Here's how the part is built. I have some questions about the finished solid (model axes, mm). Face numbers are marked on the shaded views. Round coordinates to 2 decimals unless told otherwise and drop trailing zeros. Order: outer loops, then holes, each group sorted by start corner. A loop starts at its lowest first (then second) coordinate and runs counter-clockwise, first axis right, second up.
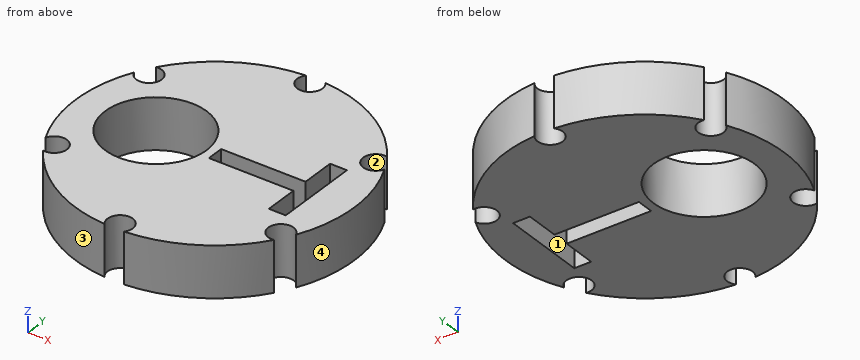
```python
from build123d import *

# Parameters (mm, degrees)
SKETCH1_R           = 16.5
BOSS_EXTRUDE1_DEPTH = 6
SKETCH2_R           = 1.5
CUT_EXTRUDE1_DEPTH  = 25.093567606
SKETCH3_R           = 6
CUT_EXTRUDE2_DEPTH  = 25.065971427
CUT_EXTRUDE3_DEPTH  = 25.065971427


with BuildPart() as part:
    # Sketch1 → Boss-Extrude1 (new body)
    with BuildSketch(Plane.XY):
        Circle(SKETCH1_R)
    extrude(amount=BOSS_EXTRUDE1_DEPTH)

    # Sketch2 → Cut-Extrude1 (cut, through all)
    with BuildSketch(Plane.XY.offset(6)):
        with Locations((0, 15.5)):
            Circle(SKETCH2_R)
        with Locations((13.423393759, 7.75)):
            Circle(SKETCH2_R)
        with Locations((13.423393759, -7.75)):
            Circle(SKETCH2_R)
        with Locations((0, -15.5)):
            Circle(SKETCH2_R)
        with Locations((-13.423393759, -7.75)):
            Circle(SKETCH2_R)
        with Locations((-13.423393759, 7.75)):
            Circle(SKETCH2_R)
    extrude(amount=-CUT_EXTRUDE1_DEPTH, mode=Mode.SUBTRACT)

    # Sketch3 → Cut-Extrude2 (cut, through all)
    with BuildSketch(Plane.XY.offset(6)):
        with Locations((-7, 0)):
            Circle(SKETCH3_R)
    extrude(amount=-CUT_EXTRUDE2_DEPTH, mode=Mode.SUBTRACT)

    # Sketch5 → Cut-Extrude3 (cut, through all)
    with BuildSketch(Plane.XY.offset(6)):
        Polygon((12, 5), (10, 5), (10, 1), (0, 1), (0, -1), (10, -1), (10, -5), (12, -5), align=None)
    extrude(amount=-CUT_EXTRUDE3_DEPTH, mode=Mode.SUBTRACT)


solid = part.part
```
1. I need wall thicknesses on probe 1 along X at (y, z) = (3, 3.9); probe 2 along Y at (x, z) = (12.5, 0.45); probe 3 along X at (y, z) = (7.75, 1.95). Which ranges of each line are inside material? Lowest first, please.
Evaluation:
probe 1: x = -16.22 to -12.2, -1.8 to 10, 12 to 16.22
probe 2: y = -10.77 to -8.93, -6.57 to 6.57, 8.93 to 10.77
probe 3: x = -11.92 to 11.92
2. I'm going to push flat-ended pins straight in: P1, Ø0.6, axis at x = 11, z = 2, coming from the +Y side; P2, Ø3, axis at x = 11.5, z = 5, coming from the +Y side. Where does each tip first touch, or does it pass through?
Evaluation:
P1: stops at y = 12.56
P2: stops at y = 13.12
3. If we section it at A-A, the plane y = 0: Write out the boundary of the cut face in (x, z), and give its area (3 significant figures).
Evaluation:
outline: (-16.5, 0) - (-13, 0) - (-13, 6) - (-16.5, 6) - close; (-1, 0) - (0, 0) - (0, 6) - (-1, 6) - close; (12, 0) - (16.5, 0) - (16.5, 6) - (12, 6) - close
area: 54.0 mm2
4. If we section it at D-D, the plane y = 15.5: Write out the boundary of the cut face in (x, z).
Evaluation:
outline: (-5.66, 0) - (-1.5, 0) - (-1.5, 6) - (-5.66, 6) - close; (1.5, 0) - (5.66, 0) - (5.66, 6) - (1.5, 6) - close
5. If we mould it in two halves opening along X, with no side actions, what happens to the marked faces 1, 2, 3 and 4? For each: released by +X, released by -X, zero draft, split by the parting line, or undercut.
Evaluation:
face 1: undercut
face 2: undercut
face 3: released by -X
face 4: released by +X
6. If we section it at C-C, the plane z = 4.05: Write out the boundary of the cut face in (x, y).
Evaluation:
outline: (-14.83, -7.23) arc R1.5 cw (long way) to (-13.68, -9.23) arc R16.5 ccw to (-1.15, -16.46) arc R1.5 cw (long way) to (1.15, -16.46) arc R16.5 ccw to (13.68, -9.23) arc R1.5 cw (long way) to (14.83, -7.23) arc R16.5 ccw to (14.83, 7.23) arc R1.5 cw (long way) to (13.68, 9.23) arc R16.5 ccw to (1.15, 16.46) arc R1.5 cw (long way) to (-1.15, 16.46) arc R16.5 ccw to (-13.68, 9.23) arc R1.5 cw (long way) to (-14.83, 7.23) arc R16.5 ccw to start; hole circle Ø12 at (-7, 0); hole (0, -1) - (10, -1) - (10, -5) - (12, -5) - (12, 5) - (10, 5) - (10, 1) - (0, 1) - close
7. If we section it at B-B, the plane x = 3: Write out the boundary of the cut face in (y, z).
Evaluation:
outline: (-16.22, 0) - (-1, 0) - (-1, 6) - (-16.22, 6) - close; (1, 0) - (16.22, 0) - (16.22, 6) - (1, 6) - close
